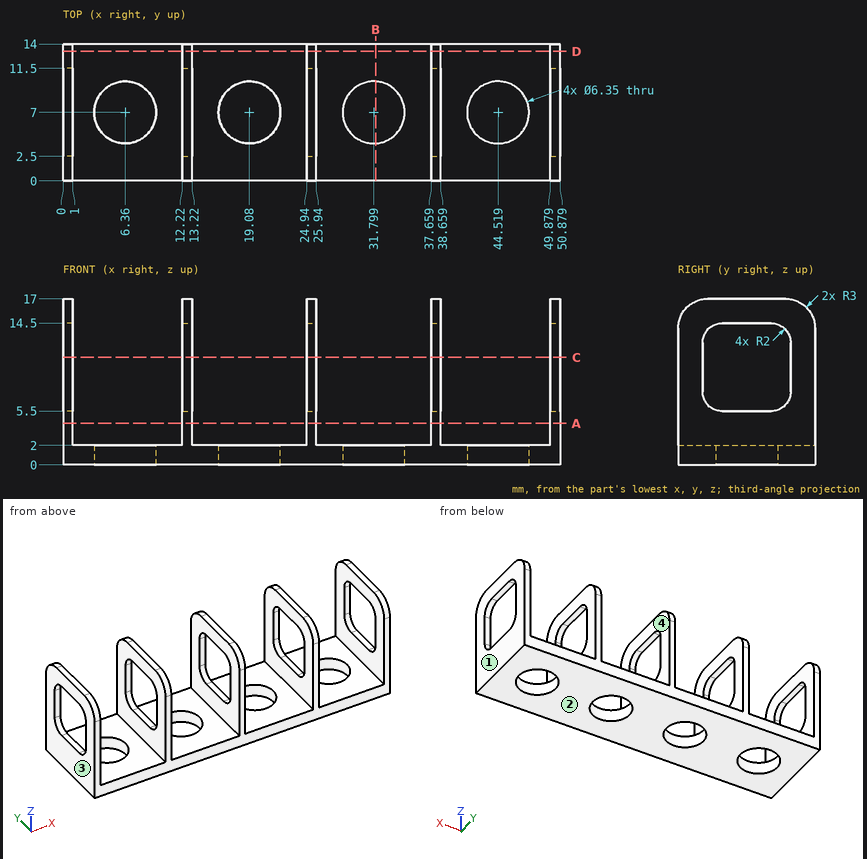
Study the drawing (mm; zero at the part's minimum x, y, z) and answer. Round coordinates to 2 decimals unless told otherwise and drop trailing zeros. Write each loop counter-clockwise with the first axis right and the second up, starting at its lowest first coordinate (ties: lowest second). Pieces come first, ordered by that corner, then holes. Notation, with made-up numbers: (-21, 76.25) - (-1, 76.25) arc R24 ccw to (-1, 113.25) - close; hole circle Ø8 at (65, -3). An arc over 180 degrees is marked (long way). Use a Markdown table: item, result. Add a question column.
1. The part is cut by section B-B (x = 32). Write down the section's boundary in (y, z).
2. The part is cut by section A-A (z = 4.25). Write down the section's boundary in (x, y).
3. The part is cut by section D-D (y = 13.25). Write down the section's boundary in (x, z) (1 decimal).
4. For a pull along X with two mould halves and no side action, classify the marked faces 1, 2, 3 and 4 as +X half, -X half, draft (parallel to the pull), parting line (faces both ways), or undercut.
5. A flat-ended cylindrical pin translates along its axis: P1, Ø6, axis at x = 31.5, y = 10.5, coming from the +Z side. Find the tip coordinate at first contact, or state that the pin passes through.
6. The part is cut by section C-C (z = 11). Give the number of separate pieces and of enclosed holes in the cut face.
7. Consider line 1 (X direction, y = 5.75, z = 3.5); line 2 (Z direction, x = 6.5, y = 10.75); line 3 (Y direction, x = 7, z = 1.25). Determine where each line is inside the solid, lowest interval first.
Reported:
| question | item | result |
|---|---|---|
| 1 | outline | (0, 0) - (3.83, 0) - (3.83, 2) - (0, 2) - close; (10.17, 0) - (14, 0) - (14, 2) - (10.17, 2) - close |
| 2 | outline | (0, 0) - (1, 0) - (1, 14) - (0, 14) - close; (12.22, 0) - (13.22, 0) - (13.22, 14) - (12.22, 14) - close; (24.94, 0) - (25.94, 0) - (25.94, 14) - (24.94, 14) - close; (37.66, 0) - (38.66, 0) - (38.66, 14) - (37.66, 14) - close; (49.88, 0) - (50.88, 0) - (50.88, 14) - (49.88, 14) - close |
| 3 | outline | (0, 0) - (50.9, 0) - (50.9, 16) - (49.9, 16) - (49.9, 2) - (38.7, 2) - (38.7, 16) - (37.7, 16) - (37.7, 2) - (25.9, 2) - (25.9, 16) - (24.9, 16) - (24.9, 2) - (13.2, 2) - (13.2, 16) - (12.2, 16) - (12.2, 2) - (1, 2) - (1, 16) - (0, 16) - close |
| 4 | face 1 | +X half |
| 4 | face 2 | draft |
| 4 | face 3 | -X half |
| 4 | face 4 | undercut |
| 5 | P1 | z = 2 |
| 6 | separate pieces | 10 |
| 6 | enclosed holes | 0 |
| 7 | line 1 | 0 to 1, 12.22 to 13.22, 24.94 to 25.94, 37.66 to 38.66, 49.88 to 50.88 |
| 7 | line 2 | 0 to 2 |
| 7 | line 3 | 0 to 3.89, 10.11 to 14 |
